from build123d import *

# Parameters (mm, degrees)
SKETCH_R     = 1.45
PAD_DEPTH    = 2
SKETCH001_W  = 51.75
SKETCH001_H  = 6
PAD001_DEPTH = 1


with BuildPart() as part:
    # Sketch → Pad (new body)
    with BuildSketch(Plane.XY):
        with BuildLine():
            Line((-29.5, 15), (29.5, 15))
            ThreePointArc((32.5, 12), (31.62132, 14.12132), (29.5, 15))
            Line((32.5, 12), (32.5, -12))
            ThreePointArc((29.5, -15), (31.62132, -14.12132), (32.5, -12))
            Line((29.5, -15), (-29.5, -15))
            ThreePointArc((-32.5, -12), (-31.62132, -14.12132), (-29.5, -15))
            Line((-32.5, -12), (-32.5, 12))
            ThreePointArc((-29.5, 15), (-31.62132, 14.12132), (-32.5, 12))
        make_face()
        with Locations((-29, 11.5)):
            Circle(SKETCH_R, mode=Mode.SUBTRACT)
        with Locations((29, 11.5)):
            Circle(SKETCH_R, mode=Mode.SUBTRACT)
        with Locations((-29, -11.5)):
            Circle(SKETCH_R, mode=Mode.SUBTRACT)
        with Locations((29, -11.5)):
            Circle(SKETCH_R, mode=Mode.SUBTRACT)
    extrude(amount=PAD_DEPTH)

    # Sketch001 (on Face14 of Pad) → Pad001 (join)
    with BuildSketch(Plane.XY.offset(2)):
        with Locations((0, 11.5)):
            Rectangle(SKETCH001_W, SKETCH001_H)
    extrude(amount=PAD001_DEPTH)


solid = part.part
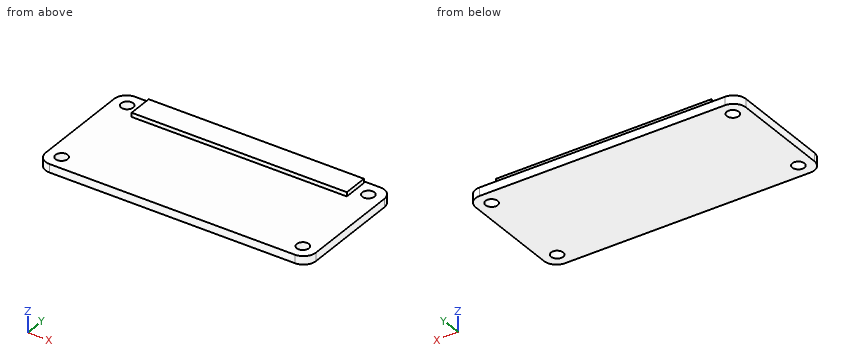
For this review, take the finished solid that the model builds, in its own axes (mm). Round coordinates to 2 decimals unless told otherwise and drop trailing zeros. Write each loop counter-clockwise with the first axis right and the second up, starting at its lowest first coordinate (ties: lowest second). Pieces come first, ordered by that corner, then holes. Notation, with made-up numbers: (85, 50) - (132, 50) arc R11 cw to (132, 58) - close; hole circle Ø10 at (80, 5.25). An arc over 180 degrees is marked (long way). Use a Markdown table: item, result.
Q1. Clearance check with flat-ended pins moving along their axes: pin 1 (0.8 mm diameter, centred on x = 11.5, z = 2.5, fed in from -Y); pin 2 (4.5 mm diameter, centred on x = -29, y = 11.5, fed in from +Z); pin 3 (0.5 mm diameter, centred on x = 11.5, z = 2.5, fed in from +Y). State where each tip first meets the part, or that it passes through.
Derived:
| item | result |
|---|---|
| pin 1 | stops at y = 8.5 |
| pin 2 | stops at z = 2 |
| pin 3 | stops at y = 14.5 |
Q2. We need section A-A (z = 0.8). Give the boundary of the cut face in (x, y), plus the area to 3 significant figures.
Derived:
| item | result |
|---|---|
| outline | (-32.5, -12) arc R3 ccw to (-29.5, -15) - (29.5, -15) arc R3 ccw to (32.5, -12) - (32.5, 12) arc R3 ccw to (29.5, 15) - (-29.5, 15) arc R3 ccw to (-32.5, 12) - close; hole circle Ø2.9 at (-29, -11.5); hole circle Ø2.9 at (-29, 11.5); hole circle Ø2.9 at (29, -11.5); hole circle Ø2.9 at (29, 11.5) |
| area | 1,920 mm2 |
Q3. Wall thickness on line 1 along Y through (x, z) = (-29, 1.25); line 2 along Z through (x, y) = (-17.5, 5); line 3 along Y through (x, z) = (15.5, 2.6): over which ranges is each line inside the solid? List them lowest first.
Derived:
| item | result |
|---|---|
| line 1 | y = -15 to -12.95, -10.05 to 10.05, 12.95 to 15 |
| line 2 | z = 0 to 2 |
| line 3 | y = 8.5 to 14.5 |
Q4. We need section C-C (y = 2.75). Give the boundary of the cut face in (x, z), plus the area to 3 significant figures.
Derived:
| item | result |
|---|---|
| outline | (-32.5, 0) - (32.5, 0) - (32.5, 2) - (-32.5, 2) - close |
| area | 130 mm2 |
Q5. We need section B-B (x = -16.5). Give the boundary of the cut face in (y, z), plus the area to 3 significant figures.
Derived:
| item | result |
|---|---|
| outline | (-15, 0) - (15, 0) - (15, 2) - (14.5, 2) - (14.5, 3) - (8.5, 3) - (8.5, 2) - (-15, 2) - close |
| area | 66.0 mm2 |
